Part model, mm, in its own coordinate system. Face numbers are marked on the shaded views. Round coordinates to 2 decimals unless told otherwise and drop trailing zeros. Loops run counter-clockwise (first coordinate to the right, second up) from the corner with the lowest first, then second, coordinate; pieces in that order, holes last. Notation, with made-up numbers: M 20.5,83 L 52.5,83 A18 cw 52.5,108 Z; hole C 39,-2.5 d6. An arc over 180 degrees is marked long. Put each result on its own line as item: value. Start each with the question number.
1) Pull direction Z, two halves, no side cores. Call the marked faces 1 and 2: +Z half, -Z half, draft (parallel to the pull), parting line (faces both ways), or undercut.
2) Probe line 1 along X through (y, z) = (-4, 0); line 2 along X through (y, z) = (31, 0); line 3 along Z through (x, y) = (-15.5, -4.5). List the from-to ranges inside material, lowest first.
3) Slice it at C-C on y = 10. Give the cut face in (x, z), then the cut area to 3 significant figures.
4) Drop flat-ended pins along their axis: pin 1 Ø12 at (y, z) = (11, 45) entering from -X; pin 2 Ø2 at (y, z) = (20, 28) entering from +X; pin 3 Ø6 at (y, z) = (8.5, 40.5) entering from +X. Give the stop position or say it passes through.
5) Slice it at A-A on z = 0. Give the cut face in (x, y).
6) Slice it at B-B on x = 0. Give the cut face in (y, z), then the cut area to 3 significant figures.
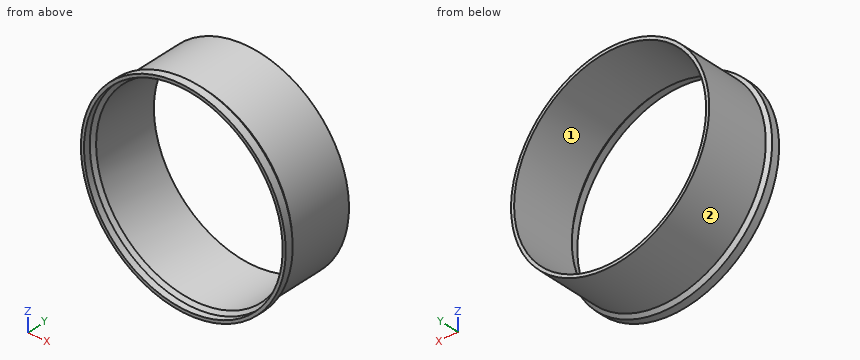
```python
from build123d import *

# Parameters (mm, degrees)
SKETCH1_R           = 77.4
SKETCH1_R_2         = 75
BOSS_EXTRUDE1_DEPTH = 50


with BuildPart() as part:
    # Sketch1 → Boss-Extrude1 (new body)
    with BuildSketch(Plane(origin=(0, 0, 0), x_dir=(1, 0, 0), z_dir=(0, 1, 0))):
        with Locations(Location((0, 0, 0), (0, 0, 270))):
            Circle(SKETCH1_R)
        with Locations(Location((0, 0, 0), (0, 0, 270))):
            Circle(SKETCH1_R_2, mode=Mode.SUBTRACT)
    extrude(amount=BOSS_EXTRUDE1_DEPTH)

    # Sketch4 → Revolve1 (revolve)
    with BuildSketch(Plane.XY, mode=Mode.PRIVATE) as revolve1_sk:
        Polygon((75, 0), (77.6, -2.6), (77.6, -7.6), (80, -7.6), (80, -1.60588745), (77.4, 0.99411255), (77.4, 0), align=None)
    revolve(revolve1_sk.sketch.rotate(Axis((0, 0, 0), (0, 1, 0)), 90), axis=Axis((0, 0, 0), (0, 1, 0)))


solid = part.part
```
Recorded:
1. face 1: undercut
1. face 2: parting line
2. line 1: x = -80 to -77.6, 77.6 to 80
2. line 2: x = -77.4 to -75, 75 to 77.4
2. line 3: z = -78.48 to -76.04, 76.04 to 78.48
3. outline: C 0,0 d154.8; hole C 0,0 d150
3. area: 1,150 mm2
4. pin 1: stops at x = -66.86
4. pin 2: stops at x = 72.54
4. pin 3: stops at x = 67.71
5. outline: M -80,-7.6 L -77.6,-7.6 L -77.6,-2.6 L -75,0 L -75,50 L -77.4,50 L -77.4,0.99 L -80,-1.61 Z; M 75,0 L 77.6,-2.6 L 77.6,-7.6 L 80,-7.6 L 80,-1.61 L 77.4,0.99 L 77.4,50 L 75,50 Z
6. outline: M -7.6,-80 L -1.61,-80 L 0.99,-77.4 L 50,-77.4 L 50,-75 L 0,-75 L -2.6,-77.6 L -7.6,-77.6 Z; M -7.6,77.6 L -2.6,77.6 L 0,75 L 50,75 L 50,77.4 L 0.99,77.4 L -1.61,80 L -7.6,80 Z
6. area: 282 mm2
